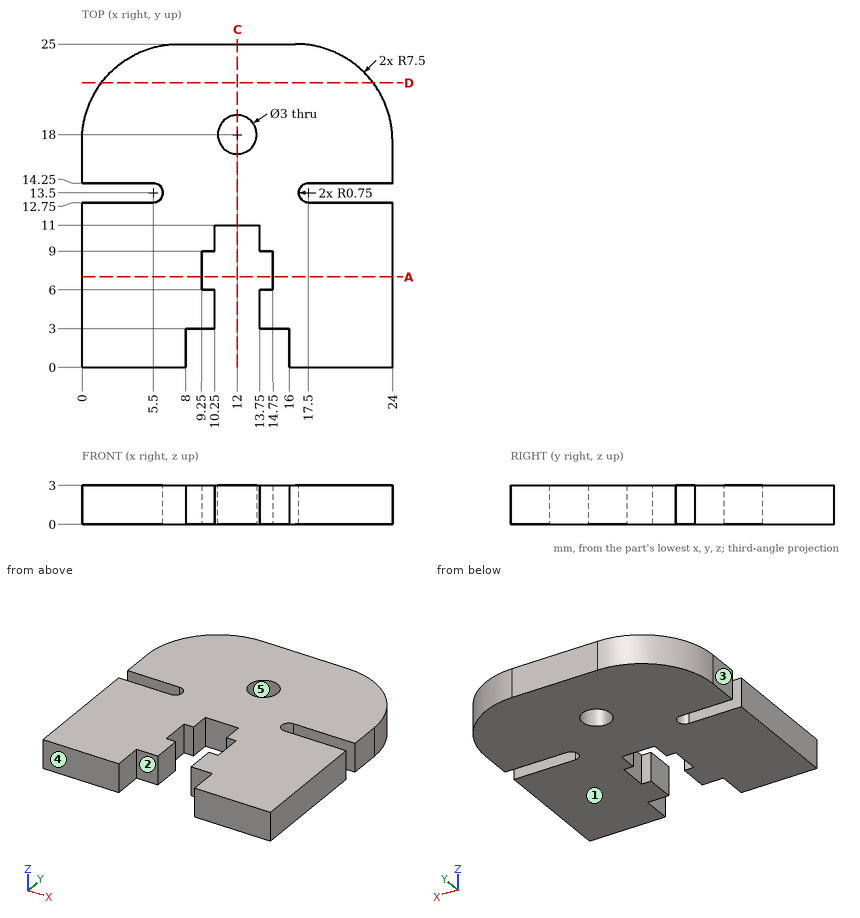
Geometry check sheet. Reference: drawing and pictorial views, mm from the part's lowest x, y, z. A direction names the side the tool comes from. Give positions to 0.01 mm unless a question says otherwise; leave off trailing zeros. Write each loop counter-clockwise with the first axis right and the second up, starting at its lowest first coordinate (ties: lowest second). Pieces come first, ordered by that corner, then holes. Notation, with made-up numbers: M 70.25,-18 L 119.25,-18 A17 cw 119.25,-7 Z; hole C 59.25,45 d7. An arc over 180 degrees is marked long. Use CSV: the item, a comma, the result in double quotes.
1) Go/stop test with flat-tipped pins: pin 1 Ø1.1 at (x, z) = (9.5, 1) entering from -Y; pin 2 Ø1.5 at (x, z) = (20, 2) entering from +Y; pin 3 Ø1.5 at (y, z) = (20.5, 0.5) entering from -X; pin 4 Ø1.8 at (x, y) = (12, 18) entering from -Z. Record where each tip stops, or that it passes through.
Final values:
pin 1,"y = 3"
pin 2,"y = 24.48"
pin 3,"x = 0.35"
pin 4,"through"
2) Cross-section at A-A (y = 7). Enter the section's corners in (x, z), plus the area to 3 significant figures.
Final values:
outline,"M 0,0 L 9.25,0 L 9.25,3 L 0,3 Z; M 14.75,0 L 24,0 L 24,3 L 14.75,3 Z"
area,"55.5 mm²"
3) Cross-section at C-C (x = 12). Enter the section's corners in (y, z), plus the area to 3 significant figures.
Final values:
outline,"M 11,0 L 16.5,0 L 16.5,3 L 11,3 Z; M 19.5,0 L 25,0 L 25,3 L 19.5,3 Z"
area,"33.0 mm²"
4) Access from +Z, -Z, +X, -X, +Y, -Y to the whole of each face (thin tool, end or side, straight path). Record for the marked faces 1 and 2.
Final values:
face 1,"-Z, +X, -X, +Y, -Y"
face 2,"+Z, -Z, -Y"
5) Material ranges on line 1 along Y through (x, z) = (12, 0.7); line 2 along X through (y, z) = (4, 1.25); line 3 along X through (y, z) = (7.75, 2.3), recorded low to high.
Final values:
line 1,"11 to 16.5, 19.5 to 25"
line 2,"0 to 10.25, 13.75 to 24"
line 3,"0 to 9.25, 14.75 to 24"
6) Release check for a two-part mould opening along X. For the marked faces 3, 4 and 5 record: released by +X, released by -X, zero draft, split by the parting line, or undercut.
Final values:
face 3,"released by -X"
face 4,"zero draft"
face 5,"undercut"
7) Cross-section at D-D (y = 22). Enter the section's corners in (x, z), plus the area to 3 significant figures.
Final values:
outline,"M 1.5,0 L 22.5,0 L 22.5,3 L 1.5,3 Z"
area,"63.0 mm²"
